The model under review builds one solid part; all positions refer to its coordinate system, in mm. Coordinates: 2 decimals unless noted, no trailing zeros. Write each loop counter-clockwise with the first axis right and the second up, starting at its lowest first coordinate (ties: lowest second). Pieces come first, ordered by that corner, then holes. Notation, with made-up numbers: (43, -5) - (92, -5) arc R17 cw to (92, 16) - close; hole circle Ø5 at (87, 20). An arc over 180 degrees is marked (long way). Put each result on its own line as item: value.
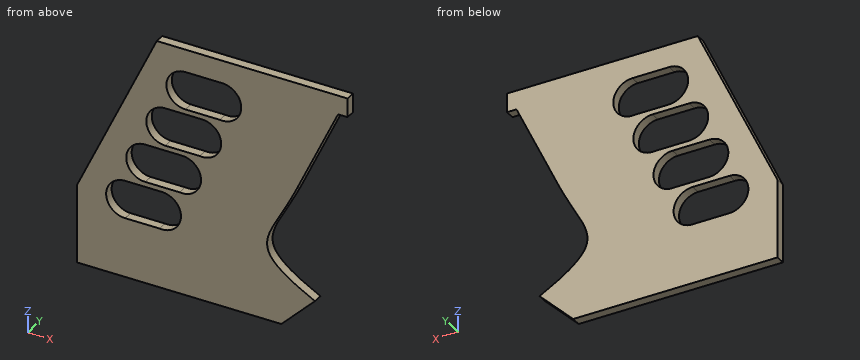
from build123d import *

# Parameters (mm, degrees)
BOSS_EXTRUDE1_DEPTH = 5
CUT_EXTRUDE1_DEPTH  = 5
CRVPATTERN1_COUNT   = 4
CRVPATTERN1_PITCH   = 25


with BuildPart() as part:
    # Sketch1 → Boss-Extrude1 (new body)
    with BuildSketch(Plane(origin=(0, 0, 0), x_dir=(1, 0, 0), z_dir=(0, 1, 0))):
        with BuildLine():
            Line((29.424030449, 17.67766953), (-78.052582598, 17.67766953))
            Line((-78.052582598, 17.67766953), (-78.052582598, -23.77998841))
            Line((-78.052582598, -23.77998841), (-36.084893364, -113.77998841))
            Line((-36.084893364, -113.77998841), (64.252030054, -113.77998841))
            Line((64.252030054, -113.77998841), (64.252030054, -103.77998841))
            Line((64.252030054, -103.77998841), (59.252030054, -103.77998841))
            Line((59.252030054, -103.77998841), (37.104377349, -56.284193911))
            add(Edge.make_bspline(
                [(47.101699979, 0), (7.916375449, -20.532992836), (22.607602938, -25.195760862), (37.104377349, -56.284193911)],
                knots=[0, 0, 0, 0, 1, 1, 1, 1], degree=3))
            Line((47.101699979, 0), (29.424030449, 17.67766953))
        make_face()
    extrude(amount=BOSS_EXTRUDE1_DEPTH)

    # Sketch2 → Cut-Extrude1 (cut)
    with BuildSketch(Plane(origin=(0, 5, 0), x_dir=(1, 0, 0), z_dir=(0, 1, 0))):
        with BuildLine():
            Line((-52.71565918, -13.77998841), (-42.71565918, -13.77998841))
            Line((-42.71565918, -13.77998841), (-34.610479114, -13.77998841))
            ThreePointArc((-34.610479114, -13.77998841), (-23.370888656, -23.131095914), (-33.389506017, -33.77998841))
            Line((-33.389506017, -33.77998841), (-43.389506017, -33.77998841))
            Line((-43.389506017, -33.77998841), (-52.71565918, -33.77998841))
            ThreePointArc((-52.71565918, -33.77998841), (-62.71565918, -23.77998841), (-52.71565918, -13.77998841))
        make_face()
    cut_extrude1 = extrude(amount=-CUT_EXTRUDE1_DEPTH, mode=Mode.SUBTRACT)

    # CrvPattern1: Cut-Extrude1 ×4
    with Locations(*[Vector(0.4226182619677251, 0, 0.9063077869307863) * (i * CRVPATTERN1_PITCH) for i in range(1, CRVPATTERN1_COUNT)]):
        add(cut_extrude1, mode=Mode.SUBTRACT)


solid = part.part
1. Consider section A-A on z = 99.5. State the section outline as (x, y) points.
Determined:
outline: (-42.74, 0) - (-27.34, 0) - (-27.34, 5) - (-42.74, 5) - close; (4.64, 0) - (57.26, 0) - (57.26, 5) - (4.64, 5) - close
2. Consider section C-C on z = 70.5. State the section outline as (x, y) points.
Determined:
outline: (-56.27, 0) - (-41.49, 0) - (-41.49, 5) - (-56.27, 5) - close; (-2.33, 0) - (43.73, 0) - (43.73, 5) - (-2.33, 5) - close
3. Consider section B-B on x = -5. State the section outline as (y, z) points.
Determined:
outline: (0, -17.68) - (5, -17.68) - (5, 62.13) - (0, 62.13) - close; (0, 75.99) - (5, 75.99) - (5, 81.75) - (0, 81.75) - close; (0, 101.75) - (5, 101.75) - (5, 113.78) - (0, 113.78) - close
4. For pin 1 Ø8 at (x, z) = (-32.5, 29) entering from -Y; pin 2 Ø1.5 at (x, y) = (60.5, 2.5) entering from -Z; pin 3 Ø3 at (y, z) = (3, 61.5) entering from -X, all flat-tipped, find the tip position at first contact; note any pin that passes through.
Determined:
pin 1: passes through
pin 2: stops at z = 103.78
pin 3: stops at x = -61.16
5. Consider section D-D on y = 1.05. Give the number of separate pieces and of enclosed holes in the cut face, plus the area to 3 significant figures.
Determined:
separate pieces: 1
enclosed holes: 4
area: 10,800 mm^2
6. To check wall thickness, follow probe 1 along Z at (x, y) = (-10, 3.55); probe 2 along Z at (x, y) = (-47, 3); probe 3 along Z at (x, y) = (-38.5, 2.5). State the ranges of each line that lie inside material, in increasing order.
Determined:
probe 1: z = -17.68 to 59.28, 78.84 to 81.75, 101.75 to 113.78
probe 2: z = -17.68 to 13.78, 33.78 to 37.69, 55.18 to 90.37
probe 3: z = -17.68 to 13.78, 33.78 to 36.44, 56.44 to 61.87, 76.32 to 108.6
